Answer from the drawing. Dimensions are ordinates in mm from the lowest x, y and z of the part. A direction names the side the tool comes from. Coordinates: 2 decimals unless noted, no trailing zeros. Write each loop counter-clockwise with the first axis right and the second up, starting at its lowest first coordinate (ties: lowest second). Pieces come first, ordered by that corner, then holes. Notation, with made-up numbers: (75.5, 20) -> (85.5, 20) arc R18 ccw to (85.5, 50) -> close; hole circle Ø8 at (63, 81). An arc over 180 degrees is marked (long way). Use CSV: the item, a comma, the result in double quotes.
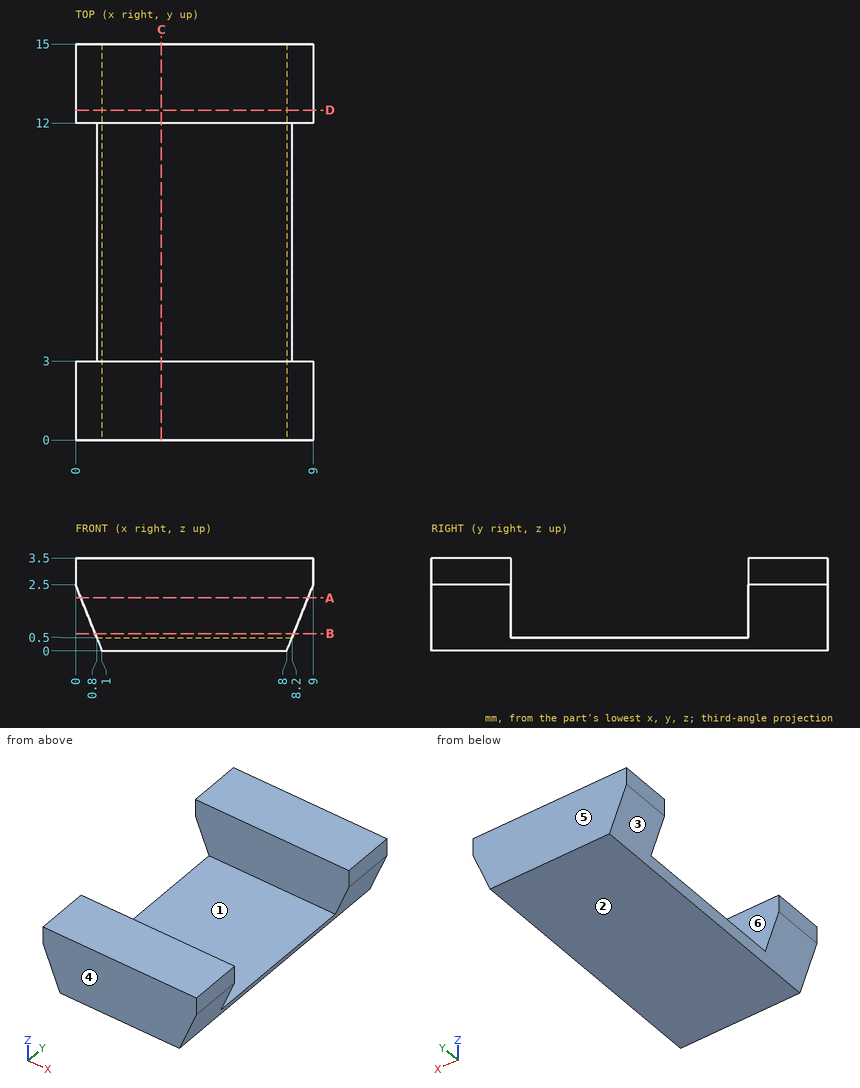
1. A cutting plane is placed at D-D (y = 12.5). Give the vertices of the cut face in (x, z), and give its area (3 significant figures).
Solutions:
outline,"(0, 2.5) -> (1, 0) -> (8, 0) -> (9, 2.5) -> (9, 3.5) -> (0, 3.5) -> close"
area,"29.0 mm^2"
2. Find the intervals of material crossed by line 1 along Y through (x, z) = (4.25, 0.8); line 2 along Z through (x, y) = (2.5, 10); line 3 along X through (y, z) = (12.5, 0.75), in increasing order.
Solutions:
line 1,"y = 0 to 3, 12 to 15"
line 2,"z = 0 to 0.5"
line 3,"x = 0.7 to 8.3"
3. For a pull along Y with two mould halves and no side action, classify the marked faces 3, 4, 5 and 6 as pulls with the +Y half, pulls with the -Y half, needs draft (parallel to the pull), parting line crosses it, or undercut.
Solutions:
face 3,"needs draft"
face 4,"pulls with the -Y half"
face 5,"pulls with the +Y half"
face 6,"undercut"
4. A cutting plane is placed at C-C (x = 3.25). Give the vertices of the cut face in (y, z), and give its area (3 significant figures).
Solutions:
outline,"(0, 0) -> (15, 0) -> (15, 3.5) -> (12, 3.5) -> (12, 0.5) -> (3, 0.5) -> (3, 3.5) -> (0, 3.5) -> close"
area,"25.5 mm^2"
5. Each of these flat-tipped pins is pushed along its axis until it touches: pin 1 Ø1.5 at (x, y) = (5.5, 4) entering from -Z; pin 2 Ø3.5 at (x, y) = (6, 8.5) entering from +Z. Where does it stop, or does it pass through?
Solutions:
pin 1,"stops at z = 0"
pin 2,"stops at z = 0.5"
6. A tool of negligible diameter and unlimited length cuts with its end or side. For the marked faces 1 and 2, from which of +Z, -Z, +X, -X, +Y, -Y can it reach the whole face along a straight path? Write none if from no direction.
Solutions:
face 1,"+Z, +X, -X"
face 2,"-Z, +X, -X, +Y, -Y"
7. A cutting plane is placed at A-A (z = 2). Give the vertices of the cut face in (x, y).
Solutions:
outline,"(0.2, 0) -> (8.8, 0) -> (8.8, 3) -> (0.2, 3) -> close; (0.2, 12) -> (8.8, 12) -> (8.8, 15) -> (0.2, 15) -> close"
8. A cutting plane is placed at B-B (z = 0.65). Give the vertices of the cut face in (x, y), and give its area (3 significant figures).
Solutions:
outline,"(0.74, 0) -> (8.26, 0) -> (8.26, 3) -> (0.74, 3) -> close; (0.74, 12) -> (8.26, 12) -> (8.26, 15) -> (0.74, 15) -> close"
area,"45.1 mm^2"
